Read the model definition and answer for the solid it produces. Units are mm, in the model's axes. Face numbers are marked on the shaded views. A direction names the side the tool comes from. Give positions to 0.01 mm unless a question says otherwise; leave off trailing zeros. Loops run counter-clockwise (first coordinate to the right, second up) from the corner with the lowest first, then second, coordinate; pieces in that order, holes last. Notation, with made-up numbers: (15.5, 75) - (43.5, 75) arc R20 ccw to (43.5, 96) - close; hole circle Ø3 at (25.25, 66.5). An arc over 180 degrees is marked (long way). Write item = value, one per line.
```python
from build123d import *

# Parameters (mm, degrees)
SKETCH_1_W               = 56
SKETCH_1_H               = 72
EXTRUDE_1_DEPTH          = 5
SHELL_1_T                = -1.5
EXTRUDE_2_DEPTH          = 5
EXTRUDE_4_REACH          = 93.351
SKETCH_11_W              = 3.2
SKETCH_11_H              = 28
CUT_EXTRUDE_1_REACH      = 93.351
SKETCH_2_7_R             = 1.05
SKETCH_2_8_R             = 1.7
CUT_EXTRUDE_2_DEPTH      = 2.5
EXTRUDE_3_DEPTH          = 1.5
CUT_EXTRUDE_3_REACH      = 93.875
SKETCH_10_3_W            = 12
SKETCH_10_3_H            = 1.5
CUT_EXTRUDE_4_DEPTH      = 92.874914966
CUT_EXTRUDE_4_DEPTH_BACK = 1
SKETCH_10_4_W            = 5
SKETCH_10_4_H            = 1
CUT_EXTRUDE_5_REACH      = 93.875
CUT_EXTRUDE_START        = -54.5
CUT_EXTRUDE_6_DEPTH      = 54.5
FILLET_1_R               = 4
FILLET_2_R               = 4
FILLET_3_R               = 1


with BuildPart() as part:
    # 草图1 → 凸台-拉伸1 (new body)
    with BuildSketch(Plane.XY):
        with Locations((-28, 36)):
            Rectangle(SKETCH_1_W, SKETCH_1_H)
    extrude(amount=EXTRUDE_1_DEPTH)

    # 抽壳1
    shell_1_openings = [part.faces().sort_by_distance(p)[0] for p in [
        (-28, 36, 5),
    ]]
    offset(amount=SHELL_1_T, openings=shell_1_openings, kind=Kind.INTERSECTION)

    # 草图2 → 凸台-拉伸2 (add)
    with BuildSketch(Plane.XY):
        with BuildLine():
            Line((0, 72), (0, 68))
            ThreePointArc((0, 68), (-0.394448725, 66.267949192), (-1.5, 64.877501001))
            Line((-1.5, 64.877501001), (-1.5, 64))
            Line((-1.5, 64), (-4, 64))
            ThreePointArc((-4, 64), (-6, 64.535898385), (-7.464101615, 66))
            Line((-7.464101615, 66), (-48.535898385, 66))
            ThreePointArc((-48.535898385, 66), (-50, 64.535898385), (-52, 64))
            Line((-52, 64), (-54.5, 64))
            Line((-54.5, 64), (-54.5, 64.877501001))
            ThreePointArc((-54.5, 64.877501001), (-55.605551275, 66.267949192), (-56, 68))
            Line((-56, 68), (-56, 72))
            Line((-56, 72), (0, 72))
        make_face()
    extrude(amount=EXTRUDE_2_DEPTH)

    # 草图11 → 凸台-拉伸4 (add, up to next)
    with BuildSketch(Plane(origin=(0, 0, 0), x_dir=(0, 0, -1), z_dir=(1, 0, 0)), mode=Mode.PRIVATE) as extrude_4_sk1:
        with Locations((-1.6, 58)):
            Rectangle(SKETCH_11_W, SKETCH_11_H)
    extrude_4_tool1 = extrude(extrude_4_sk1.sketch, amount=-EXTRUDE_4_REACH, mode=Mode.PRIVATE) - part.part
    add(extrude_4_tool1.solids().sort_by_distance((0, 58, 1.6))[0])

    # 草图2<7> → 切除-拉伸1 (cut, up to next)
    with BuildSketch(Plane.XY, mode=Mode.PRIVATE) as cut_extrude_1_sk1:
        with Locations((-52, 68)):
            Circle(SKETCH_2_7_R)
    cut_extrude_1_tool1 = extrude(cut_extrude_1_sk1.sketch, amount=CUT_EXTRUDE_1_REACH, mode=Mode.PRIVATE) & part.part
    # 草图2<7> → 切除-拉伸1 (cut, up to next)
    with BuildSketch(Plane.XY, mode=Mode.PRIVATE) as cut_extrude_1_sk2:
        with Locations(Location((-4, 68, 0), (0, 0, 180))):
            Circle(SKETCH_2_7_R)
    cut_extrude_1_tool2 = extrude(cut_extrude_1_sk2.sketch, amount=CUT_EXTRUDE_1_REACH, mode=Mode.PRIVATE) & part.part
    add(cut_extrude_1_tool1.solids().sort_by_distance((-52, 68, 0))[0], mode=Mode.SUBTRACT)
    add(cut_extrude_1_tool2.solids().sort_by_distance((-4, 68, 0))[0], mode=Mode.SUBTRACT)

    # 草图2<8> → 切除-拉伸2 (cut)
    with BuildSketch(Plane.XY):
        with Locations((-52, 68)):
            Circle(SKETCH_2_8_R)
        with Locations(Location((-4, 68, 0), (0, 0, 180))):
            Circle(SKETCH_2_8_R)
    extrude(amount=CUT_EXTRUDE_2_DEPTH, mode=Mode.SUBTRACT)

    # 草图10 → 凸台-拉伸3 (add)
    with BuildSketch(Plane.XZ):
        with BuildLine():
            Line((-40, 5), (-40, 8))
            Line((-40, 8), (-52, 8))
            Line((-52, 8), (-52, 11))
            Line((-52, 11), (-34, 11))
            ThreePointArc((-34, 11), (-29.757359313, 9.242640687), (-28, 5))
            Line((-28, 5), (-40, 5))
        make_face()
    extrude(amount=-EXTRUDE_3_DEPTH)

    # 草图10<3> → 切除-拉伸3 (cut, up to next)
    with BuildSketch(Plane.XZ, mode=Mode.PRIVATE) as cut_extrude_3_sk1:
        with Locations((-14.2, 2.25)):
            Rectangle(SKETCH_10_3_W, SKETCH_10_3_H)
    cut_extrude_3_tool1 = extrude(cut_extrude_3_sk1.sketch, amount=-CUT_EXTRUDE_3_REACH, mode=Mode.PRIVATE) & part.part
    add(cut_extrude_3_tool1.solids().sort_by_distance((-14.2, 0, 2.25))[0], mode=Mode.SUBTRACT)

    # 草图10<4> → 切除-拉伸4 (cut, two sides: drawn at the far end of the back side and taken through both)
    with BuildSketch(Plane.XZ.offset(-CUT_EXTRUDE_4_DEPTH_BACK)):
        with Locations((-14.2, 1)):
            Rectangle(SKETCH_10_4_W, SKETCH_10_4_H)
    extrude(amount=CUT_EXTRUDE_4_DEPTH + CUT_EXTRUDE_4_DEPTH_BACK, mode=Mode.SUBTRACT)

    # 草图8 → 切除-拉伸5 (cut, up to next)
    with BuildSketch(Plane.ZY.offset(56), mode=Mode.PRIVATE) as cut_extrude_5_sk1:
        with BuildLine():
            Line((2.5, 38.500900756), (2.5, 12.087099244))
            ThreePointArc((2.5, 12.087099244), (3.18337521, 9.851031266), (5, 8.379))
            Line((5, 8.379), (5, 42.209))
            ThreePointArc((5, 42.209), (3.18337521, 40.736968734), (2.5, 38.500900756))
        make_face()
    cut_extrude_5_tool1 = extrude(cut_extrude_5_sk1.sketch, amount=-CUT_EXTRUDE_5_REACH, mode=Mode.PRIVATE) & part.part
    add(cut_extrude_5_tool1.solids().sort_by_distance((-56, 25.294, 3.786685))[0], mode=Mode.SUBTRACT)

    # 草图9 → 切除-拉伸6 (cut)
    with BuildSketch(Plane(origin=(0, 0, 0), x_dir=(0, 0, -1), z_dir=(1, 0, 0)).offset(CUT_EXTRUDE_START)):
        with BuildLine():
            Line((-1.5, 41), (-1.5, 51))
            ThreePointArc((-1.5, 51), (-7, 56.5), (-12.5, 51))
            Line((-12.5, 51), (-12.5, 41))
            ThreePointArc((-12.5, 41), (-7, 35.5), (-1.5, 41))
        make_face()
    extrude(amount=CUT_EXTRUDE_6_DEPTH, mode=Mode.SUBTRACT)

    # 圆角1
    fillet_1_edges = [part.edges().sort_by_distance(p)[0] for p in [
        (0, 0, 2.5),
        (-56, 0, 2.5),
        (-56, 72, 2.5),
        (0, 72, 2.5),
    ]]
    fillet(fillet_1_edges, radius=FILLET_1_R)

    # 圆角2
    fillet_2_edges = [part.edges().sort_by_distance(p)[0] for p in [
        (-1.5, 1.5, 3.25),
        (-54.5, 1.5, 3.25),
    ]]
    fillet(fillet_2_edges, radius=FILLET_2_R)

    # 圆角3
    # the kernel refuses this fillet: 1 mm, written as the material it takes off along each edge
    with BuildSketch(Plane(origin=(-52, 68, 0), x_dir=(1, 0, 0), z_dir=(0, -1, 0))) as fillet_3_piece_1:
        with BuildLine():
            CenterArc((1.7 + FILLET_3_R, FILLET_3_R), FILLET_3_R, 180, 90)
            Line((1.7, FILLET_3_R), (1.7, 0))
            Line((1.7, 0), (1.7 + FILLET_3_R, 0))
        make_face()
    revolve(axis=Axis((-52, 68, 0), (0, 0, 1)), mode=Mode.SUBTRACT)
    with BuildSketch(Plane(origin=(-4, 68, 0), x_dir=(-1, 0, 0), z_dir=(0, 1, 0))) as fillet_3_piece_2:
        with BuildLine():
            CenterArc((1.7 + FILLET_3_R, FILLET_3_R), FILLET_3_R, 180, 90)
            Line((1.7, FILLET_3_R), (1.7, 0))
            Line((1.7, 0), (1.7 + FILLET_3_R, 0))
        make_face()
    revolve(axis=Axis((-4, 68, 0), (0, 0, 1)), mode=Mode.SUBTRACT)
    with BuildSketch(Plane(origin=(-4, 4, 0), x_dir=(0, -1, 0), z_dir=(-1, 0, 0))) as fillet_3_piece_3:
        with BuildLine():
            CenterArc((4 - FILLET_3_R, FILLET_3_R), FILLET_3_R, 270, 90)
            Line((4 - FILLET_3_R, 0), (4, 0))
            Line((4, 0), (4, FILLET_3_R))
        make_face()
    revolve(axis=Axis((-4, 4, 0), (0, 0, 1)), revolution_arc=90, mode=Mode.SUBTRACT)
    with BuildSketch(Plane(origin=(0, 4, 0), x_dir=(0, 0, 1), z_dir=(0, 1, 0))) as fillet_3_piece_4:
        with BuildLine():
            CenterArc((FILLET_3_R, -FILLET_3_R), FILLET_3_R, 90, 90)
            Line((0, -FILLET_3_R), (0, 0))
            Line((0, 0), (FILLET_3_R, 0))
        make_face()
    extrude(amount=64, mode=Mode.SUBTRACT)
    with BuildSketch(Plane(origin=(-4, 68, 0), x_dir=(0, 1, 0), z_dir=(-1, 0, 0))) as fillet_3_piece_5:
        with BuildLine():
            CenterArc((4 - FILLET_3_R, -FILLET_3_R), FILLET_3_R, 0, 90)
            Line((4, -FILLET_3_R), (4, 0))
            Line((4, 0), (4 - FILLET_3_R, 0))
        make_face()
    revolve(axis=Axis((-4, 68, 0), (0, 0, -1)), revolution_arc=90, mode=Mode.SUBTRACT)
    with BuildSketch(Plane(origin=(-52, 72, 0), x_dir=(0, -1, 0), z_dir=(1, 0, 0))) as fillet_3_piece_6:
        with BuildLine():
            CenterArc((FILLET_3_R, -FILLET_3_R), FILLET_3_R, 90, 90)
            Line((0, -FILLET_3_R), (0, 0))
            Line((0, 0), (FILLET_3_R, 0))
        make_face()
    extrude(amount=48, mode=Mode.SUBTRACT)
    with BuildSketch(Plane(origin=(-52, 68, 0), x_dir=(0, 1, 0), z_dir=(1, 0, 0))) as fillet_3_piece_7:
        with BuildLine():
            CenterArc((4 - FILLET_3_R, FILLET_3_R), FILLET_3_R, 270, 90)
            Line((4, FILLET_3_R), (4, 0))
            Line((4, 0), (4 - FILLET_3_R, 0))
        make_face()
    revolve(axis=Axis((-52, 68, 0), (0, 0, 1)), revolution_arc=90, mode=Mode.SUBTRACT)
    with BuildSketch(Plane(origin=(-56, 68, 0), x_dir=(1, 0, 0), z_dir=(0, -1, 0))) as fillet_3_piece_8:
        with BuildLine():
            CenterArc((FILLET_3_R, FILLET_3_R), FILLET_3_R, 180, 90)
            Line((0, FILLET_3_R), (0, 0))
            Line((0, 0), (FILLET_3_R, 0))
        make_face()
    extrude(amount=64, mode=Mode.SUBTRACT)
    with BuildSketch(Plane(origin=(-52, 4, 0), x_dir=(0, -1, 0), z_dir=(1, 0, 0))) as fillet_3_piece_9:
        with BuildLine():
            CenterArc((4 - FILLET_3_R, -FILLET_3_R), FILLET_3_R, 0, 90)
            Line((4, -FILLET_3_R), (4, 0))
            Line((4, 0), (4 - FILLET_3_R, 0))
        make_face()
    revolve(axis=Axis((-52, 4, 0), (0, 0, -1)), revolution_arc=90, mode=Mode.SUBTRACT)
    with BuildSketch(Plane(origin=(-4, 0, 0), x_dir=(0, 0, 1), z_dir=(-1, 0, 0))) as fillet_3_piece_10:
        with BuildLine():
            CenterArc((FILLET_3_R, FILLET_3_R), FILLET_3_R, 180, 90)
            Line((0, FILLET_3_R), (0, 0))
            Line((0, 0), (FILLET_3_R, 0))
        make_face()
    extrude(amount=48, mode=Mode.SUBTRACT)


solid = part.part
```
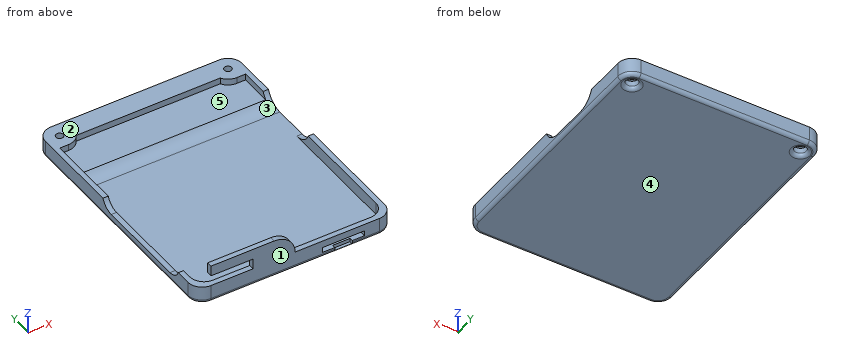
1) The mould has two halves that part along X. Classify the marked faces 4 and 5: pulls with the +X half, pulls with the -X half, needs draft (parallel to the pull), parting line crosses it, or undercut.
Output:
face_4 = needs draft
face_5 = undercut
2) Find the intervals of material crossed by probe 1 along X at (y, z) = (68, 2.1); probe 2 along X at (y, z) = (68, 3.45); probe 3 along Y at (x, z) = (-52, 4.2), in increasing order.
Output:
probe_1 = -56 to -53.7, -50.3 to -5.7, -2.3 to 0
probe_2 = -56 to -53.05, -50.95 to -5.05, -2.95 to 0
probe_3 = 0 to 1.79, 64 to 66.95, 69.05 to 72
3) A cutting plane is placed at D-D on z = 6.75. Determine the outline of the cut face in (x, y), then the cut area to 3 significant figures.
Output:
outline = (-40, 0) - (-28.26, 0) - (-28.26, 1.5) - (-40, 1.5) - close
area = 17.6 mm²
4) Each of these flat-tipped pins is pushed along its axis until it touches: P1, Ø12, axis at x = -36.5, y = 61, coming from the +Z side; P2, Ø1.7, axis at x = -4, y = 68.5, coming from the -Z side; P3, Ø1, axis at x = -9.5, y = 11.5, coming from the +Z side; P4, Ø4, axis at y = 40.5, z = 8.5, coming from the -X side. Where does it stop, or does it pass through?
Output:
P1 = 5
P2 = 2.5
P3 = 1.5
P4 = through
5) A cutting plane is placed at C-C on x = -26. Determine the outline of the cut face in (y, z).
Output:
outline = (0, 1) arc R1 ccw to (1, 0) - (71, 0) arc R1 ccw to (72, 1) - (72, 5) - (66, 5) - (66, 3.2) - (54.98, 3.2) arc R5.5 cw to (51, 1.5) - (1.5, 1.5) - (1.5, 5) - (0, 5) - close
6) A tool of negligible diameter and unlimited length cuts with its end or side. For the marked faces 1, 2 and 3, from which of +Z, -Z, +X, -X, +Y, -Y can it reach the whole face along a straight path? Write none if from no direction.
Output:
face_1 = +Z, -Z, +X, -X, -Y
face_2 = +Z, +X, -X, +Y
face_3 = +Z, +X
7) A cutting plane is placed at B-B on y = 32.5. Determine the outline of the cut face in (x, z).
Output:
outline = (-56, 1) arc R1 ccw to (-55, 0) - (-1, 0) arc R1 ccw to (0, 1) - (0, 5) - (-1.5, 5) - (-1.5, 1.5) - (-54.5, 1.5) - (-54.5, 2.5) - (-56, 2.5) - close
8) A cutting plane is placed at A-A on x = -13. Determine the outline of the cut face in (y, z), then the cut area to 3 significant figures.
Output:
outline = (0, 3) - (1.5, 3) - (1.5, 5) - (0, 5) - close; (0.13, 0.5) arc R1 ccw to (1, 0) - (71, 0) arc R1 ccw to (72, 1) - (72, 5) - (66, 5) - (66, 3.2) - (54.98, 3.2) arc R5.5 cw to (51, 1.5) - (1, 1.5) - (1, 0.5) - close
area = 151 mm²
